```python
from build123d import *

# Parameters (mm, degrees)
BOSS_EXTRUDE1_DEPTH = 160
SHELL1_START        = -80
SHELL1_OUTLINE_W    = 80
SHELL1_OUTLINE_H    = 150
SHELL1_DEPTH        = 80
SHELL1_START_2      = -100
SHELL1_2_OUTLINE_W  = 59
SHELL1_2_OUTLINE_H  = 150
SHELL1_2_DEPTH      = 20
SKETCH2_W           = 5
SKETCH2_H           = 5
CUT_EXTRUDE1_DEPTH  = 150
FILLET1_R           = 5
SKETCH4_W           = 10
SKETCH4_H           = 20
CUT_EXTRUDE2_DEPTH  = 10


# Read off the part's stored shape, not the designer's step: Shell1
with BuildPart() as part:
    # Sketch1 → Boss-Extrude1 (new body)
    with BuildSketch(Plane(origin=(0, 0, 0), x_dir=(1, 0, 0), z_dir=(0, 1, 0))):
        Polygon((50, 0), (-50, 0), (-50, 90), (-39.5, 90), (-39.5, 95), (-44.5, 95), (-44.5, 100), (44.5, 100), (44.5, 95), (39.5, 95), (39.5, 90), (50, 90), align=None)
    extrude(amount=BOSS_EXTRUDE1_DEPTH)

    # Shell1 outline → Shell1 (cut)
    with BuildSketch(Plane.XY.offset(SHELL1_START)):
        with Locations((0, 85)):
            Rectangle(SHELL1_OUTLINE_W, SHELL1_OUTLINE_H)
    extrude(amount=SHELL1_DEPTH, mode=Mode.SUBTRACT)

    # Shell1 2 outline → Shell1 2 (cut)
    with BuildSketch(Plane.XY.offset(SHELL1_START_2)):
        with Locations((0, 85)):
            Rectangle(SHELL1_2_OUTLINE_W, SHELL1_2_OUTLINE_H)
    extrude(amount=SHELL1_2_DEPTH, mode=Mode.SUBTRACT)

    # Sketch2 → Cut-Extrude1 (cut)
    with BuildSketch(Plane(origin=(0, 160, 0), x_dir=(1, 0, 0), z_dir=(0, 1, 0))):
        with Locations((-42.5, 7.5)):
            Rectangle(SKETCH2_W, SKETCH2_H)
        with Locations((42.5, 7.5)):
            Rectangle(SKETCH2_W, SKETCH2_H)
    extrude(amount=-CUT_EXTRUDE1_DEPTH, mode=Mode.SUBTRACT)

    # Fillet1
    fillet1_edges = [part.edges().sort_by_distance(p)[0] for p in [
        (45, 160, 0),
        (-45, 160, 0),
        (50, 160, -45),
        (-50, 160, -45),
        (50, 80, 0),
        (-50, 80, 0),
    ]]
    fillet(fillet1_edges, radius=FILLET1_R - 0.0001)  # a hair under: the kernel refuses the full size

    # Sketch4 → Cut-Extrude2 (cut)
    with BuildSketch(Plane(origin=(50, 0, 0), x_dir=(0, 0, -1), z_dir=(1, 0, 0))):
        with Locations((74.5, 130)):
            Rectangle(SKETCH4_W, SKETCH4_H)
    extrude(amount=-CUT_EXTRUDE2_DEPTH, mode=Mode.SUBTRACT)


solid = part.part
```
The listing builds one solid part. Answer for the finished solid, in the listing's coordinates (mm). A direction names the side the tool comes from. Coordinates: 2 decimals unless noted, no trailing zeros. Loops run counter-clockwise (first coordinate to the right, second up) from the corner with the lowest first, then second, coordinate; pieces in that order, holes last. Notation, with made-up numbers: (71.25, 29) - (127.25, 29) arc R38 ccw to (127.25, 68) - close; hole circle Ø1 at (60.5, -19). An arc over 180 degrees is marked (long way). Use a Markdown table: item, result. Add a question column.
1) The part is cut by section B-B, the plane z = -61.5. Give the vertices of the cut face in (x, y), and give its area (3 significant figures).
2) Find the intervals of material crossed by line 1 (X direction, y = 65, z = -14.5); line 2 (X direction, y = 98.5, z = -87); line 3 (Y direction, x = 38, z = -15), in increasing order.
3) The part is cut by section C-C, the plane x = -25. Give the vertices of the cut face in (y, z).
4) Given pin 1 (2.5 mm diameter, centred on y = 117.5, z = -93, fed in from +X); pin 2 (6 mm diameter, centred on x = 9.5, z = -70.5, fed in from +Y); pin 3 (2.5 mm diameter, centred on y = 75.5, z = -93, fed in from -X), each flat-ended and moving along its own axis, determine where each tip first touches the part or whether it passes through.
5) The mould has two halves that part along Y. Classify faces 1 (the flat face through (45, 130, -79.5)), 2 (the flat face through (41, 160, -64)), 3 (the flat face through (-40, 84, -3)): released by +Y, released by -Y, zero draft, split by the parting line, or undercut.
6) For faces 4 (the flat face through (44.5, 79, -98)), 5 (the flat face through (29.5, 84, -90)), 6 (the flat face through (-45, 79, -90)), determine the directions among +Z, -Z, +X, -X, +Y, -Y from which every point of the face is accessible in a straight line to the end or side of a thin tool.
Here are the results:
| question | item | result |
|---|---|---|
| 1 | outline | (-50, 0) - (50, 0) - (50, 155) arc R5 ccw to (45, 160) - (40, 160) - (40, 10) - (-40, 10) - (-40, 160) - (-45, 160) arc R5 ccw to (-50, 155) - close |
| 1 | area | 3,990 mm^2 |
| 2 | line 1 | x = -50 to -40, 40 to 50 |
| 2 | line 2 | x = -50 to -29.5, 29.5 to 50 |
| 2 | line 3 | y = 0 to 10 |
| 3 | outline | (0, -100) - (10, -100) - (10, 0) - (0, 0) - close |
| 4 | pin 1 | stops at x = 39.5 |
| 4 | pin 2 | stops at y = 10 |
| 4 | pin 3 | stops at x = -39.5 |
| 5 | face 1 | undercut |
| 5 | face 2 | released by +Y |
| 5 | face 3 | zero draft |
| 6 | face 4 | -Z, +X, +Y, -Y |
| 6 | face 5 | +Z, -Z, +Y |
| 6 | face 6 | -X, +Y, -Y |
